Could you check a few things on this drawing? It's one solid part, dimensions in mm from its lowest x, y, z. A direction names the side the tool comes from. Coordinates: 2 decimals unless noted, no trailing zeros. Order: outer loops, then holes, each group sorted by start corner. A loop starts at its lowest first (then second) coordinate and runs counter-clockwise, first axis right, second up. Notation, with made-up numbers: (-10, -39) -> (21, -39) arc R18 ccw to (21, -30) -> close; hole circle Ø4 at (32.5, 74.5). An arc over 180 degrees is marked (long way). Answer as CSV lines item,"result".
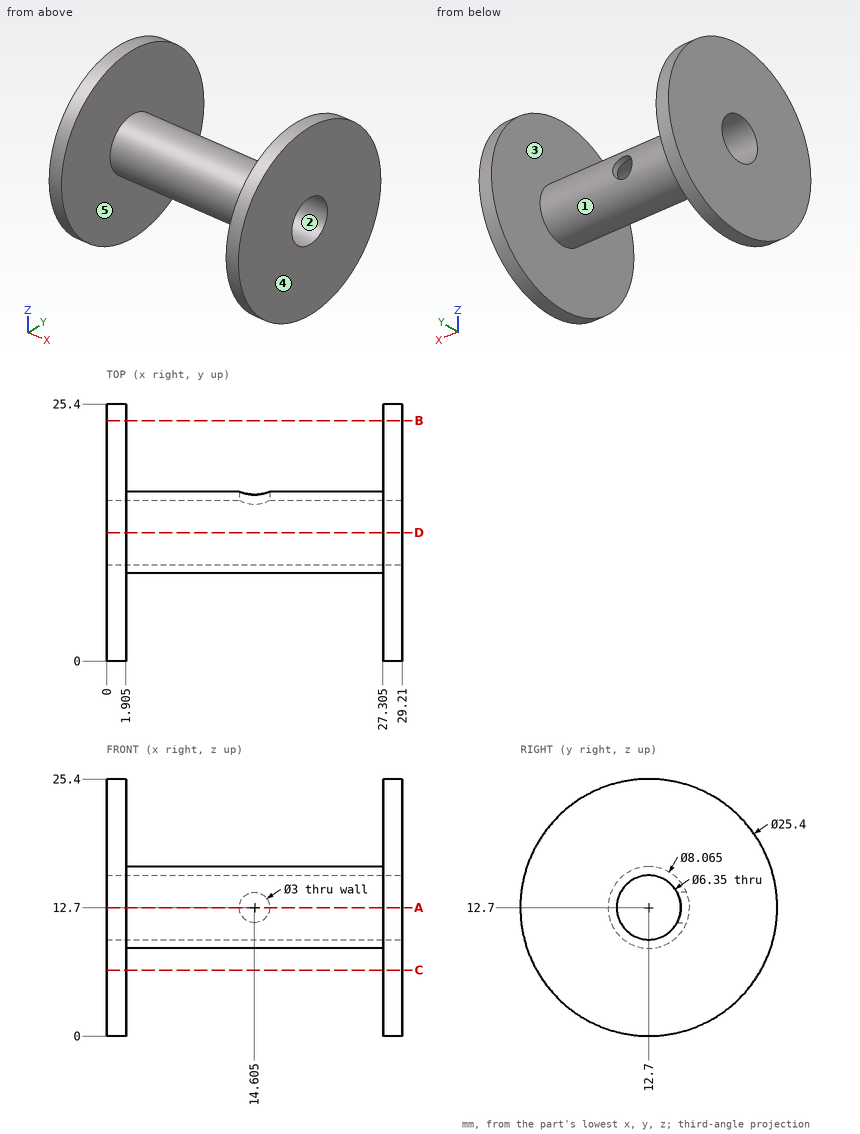
Q1. Which directions (+Z, -Z, +X, -X, +Y, -Y) give clear straight access to the entire face, cutting with the end or side of a thin tool? Please do the marked faces 4 and 5.
Solution:
face 4,"+Z, -Z, +X, +Y, -Y"
face 5,"none"
Q2. Imagine slicing it at D-D (y = 12.7). List the corners of the cut face in (x, z) for me (1 decimal), and give its area (3 significant figures).
Solution:
outline,"(0, 0) -> (1.9, 0) -> (1.9, 8.7) -> (27.3, 8.7) -> (27.3, 0) -> (29.2, 0) -> (29.2, 9.5) -> (0, 9.5) -> close; (0, 15.9) -> (29.2, 15.9) -> (29.2, 25.4) -> (27.3, 25.4) -> (27.3, 16.7) -> (1.9, 16.7) -> (1.9, 25.4) -> (0, 25.4) -> close"
area,"116 mm2"
Q3. If I drill on line 1 (X direction, y = 16.25, z = 12.7) (1 decimal); line 2 (Z direction, x = 12.75, y = 12.7) (1 decimal), over which ranges is the centre line in solid material (lowest first)?
Solution:
line 1,"0 to 13.1, 16.1 to 29.2"
line 2,"8.7 to 9.5, 15.9 to 16.7"
Q4. For P1, Ø4, axis at x = 22, y = 7.5, coming from the -Z side (1 decimal); P2, Ø5.5, axis at y = 12.7, z = 12.7, coming from the -X side; P3, Ø1.5, axis at x = 23, y = 15.5, coming from the -Z side; P4, Ø2, axis at x = 19, y = 11, coming from the +Z side, each with a flat end and sliding along its axis, tell me the tip position at first contact or that it passes through.
Solution:
P1,"z = 10.2"
P2,"through"
P3,"z = 9.23"
P4,"z = 16.67"
Q5. We'd pull the mould along Y, two halves only. Please class the marked faces 1, 2 and 3: pulls with the +Y half, pulls with the -Y half, needs draft (parallel to the pull), parting line crosses it, or undercut.
Solution:
face 1,"parting line crosses it"
face 2,"undercut"
face 3,"needs draft"
Q6. Imagine slicing it at A-A (z = 12.7). List the corners of the cut face in (x, y) for me (1 decimal).
Solution:
outline,"(0, 0) -> (1.9, 0) -> (1.9, 8.7) -> (27.3, 8.7) -> (27.3, 0) -> (29.2, 0) -> (29.2, 9.5) -> (0, 9.5) -> close; (0, 15.9) -> (13.1, 15.9) -> (13.1, 16.7) -> (1.9, 16.7) -> (1.9, 25.4) -> (0, 25.4) -> close; (16.1, 15.9) -> (29.2, 15.9) -> (29.2, 25.4) -> (27.3, 25.4) -> (27.3, 16.7) -> (16.1, 16.7) -> close"
Q7. Imagine slicing it at C-C (z = 6.5). List the corners of the cut face in (x, y) for me (1 decimal).
Solution:
outline,"(0, 1.6) -> (1.9, 1.6) -> (1.9, 23.8) -> (0, 23.8) -> close; (27.3, 1.6) -> (29.2, 1.6) -> (29.2, 23.8) -> (27.3, 23.8) -> close"
Q8. Imagine slicing it at B-B (y = 23.75). List the corners of the cut face in (x, z) for me (1 decimal).
Solution:
outline,"(0, 6.4) -> (1.9, 6.4) -> (1.9, 19) -> (0, 19) -> close; (27.3, 6.4) -> (29.2, 6.4) -> (29.2, 19) -> (27.3, 19) -> close"
